```python
from build123d import *

# Parameters (mm, degrees)
SKETCH1_W           = 7.5
SKETCH1_H           = 3.913043478
BOSS_EXTRUDE1_DEPTH = 7.5
SHELL2_T            = -0.75
SKETCH1_4_W         = 7.5
SKETCH1_4_H         = 3.913043478
BOSS_EXTRUDE2_DEPTH = 7.5
HOLE2_D             = 1.6
HOLE2_DEPTH         = 10
HOLE2_CBORE_D       = 3.5
HOLE2_CBORE_DEPTH   = 3
FILLET1_R           = 0.5


with BuildPart() as part:
    # Sketch1 → Boss-Extrude1 (new body)
    with BuildSketch(Plane.XY):
        Polygon((4, 2.086956522), (4, 6), (-4, 6), (-4, 2.086956522), (-11.5, 2.086956522), (-11.5, -2.086956522), (-4, -2.086956522), (-4, -6), (4, -6), (4, -2.086956522), (11.5, -2.086956522), (11.5, 2.086956522), align=None)
        with Locations((-7.75, 4.043478261)):
            Rectangle(SKETCH1_W, SKETCH1_H)
        with Locations((7.75, 4.043478261)):
            Rectangle(SKETCH1_W, SKETCH1_H)
        with Locations((-7.75, -4.043478261)):
            Rectangle(SKETCH1_W, SKETCH1_H)
        with Locations((7.75, -4.043478261)):
            Rectangle(SKETCH1_W, SKETCH1_H)
    extrude(amount=BOSS_EXTRUDE1_DEPTH)

    # Shell2
    shell2_openings = [part.faces().sort_by_distance(p)[0] for p in [
        (0, 0, 7.5),
    ]]
    offset(amount=SHELL2_T, openings=shell2_openings, kind=Kind.INTERSECTION)

    # Sketch1<4> → Boss-Extrude2 (add)
    with BuildSketch(Plane.XY):
        with Locations((7.75, 4.043478261)):
            Rectangle(SKETCH1_4_W, SKETCH1_4_H)
        with Locations((-7.75, 4.043478261)):
            Rectangle(SKETCH1_4_W, SKETCH1_4_H)
        with Locations((-7.75, -4.043478261)):
            Rectangle(SKETCH1_4_W, SKETCH1_4_H)
        with Locations((7.75, -4.043478261)):
            Rectangle(SKETCH1_4_W, SKETCH1_4_H)
    extrude(amount=BOSS_EXTRUDE2_DEPTH)

    # Hole2
    with Locations(Plane(origin=(0, 0, 0), x_dir=(-1, 0, 0), z_dir=(0, 0, -1))):
        with Locations((-9.9, -4), (9.9, 4), (9.9, -4), (-9.9, 4)):
            CounterBoreHole(HOLE2_D / 2, HOLE2_CBORE_D / 2, HOLE2_CBORE_DEPTH, depth=HOLE2_DEPTH)

    # Fillet1
    # the kernel refuses this fillet: 0.5 mm, written as the material it takes off along each edge
    with BuildSketch(Plane(origin=(-11.5, 6, -1.25), x_dir=(1, 0, 0), z_dir=(0, 0, 1)), Plane(origin=(11.5, -6, -1.25), x_dir=(-1, 0, 0), z_dir=(0, 0, 1))) as fillet1_piece_1:
        with BuildLine():
            CenterArc((FILLET1_R, -FILLET1_R), FILLET1_R, 90, 90)
            Line((0, -FILLET1_R), (0, 0))
            Line((0, 0), (FILLET1_R, 0))
        make_face()
    extrude(amount=10, mode=Mode.SUBTRACT)
    with BuildSketch(Plane(origin=(-11.5, 4.541127656, 0), x_dir=(1, 0, 0), z_dir=(0, -1, 0)), Plane(origin=(11.5, 4.541127656, 0), x_dir=(0, 0, 1), z_dir=(0, -1, 0))) as fillet1_piece_2:
        with BuildLine():
            CenterArc((FILLET1_R, FILLET1_R), FILLET1_R, 180, 90)
            Line((0, FILLET1_R), (0, 0))
            Line((0, 0), (FILLET1_R, 0))
        make_face()
    extrude(amount=9.082255312, mode=Mode.SUBTRACT)
    with BuildSketch(Plane(origin=(12.75, 6, 0), x_dir=(0, 0, 1), z_dir=(-1, 0, 0))) as fillet1_piece_3:
        with BuildLine():
            CenterArc((FILLET1_R, -FILLET1_R), FILLET1_R, 90, 90)
            Line((0, -FILLET1_R), (0, 0))
            Line((0, 0), (FILLET1_R, 0))
        make_face()
    extrude(amount=25.5, mode=Mode.SUBTRACT)
    with BuildSketch(Plane(origin=(11.5, 6, -1.25), x_dir=(-1, 0, 0), z_dir=(0, 0, 1)), Plane(origin=(-11.5, -6, -1.25), x_dir=(1, 0, 0), z_dir=(0, 0, 1))) as fillet1_piece_4:
        with BuildLine():
            CenterArc((FILLET1_R, FILLET1_R), FILLET1_R, 180, 90)
            Line((0, FILLET1_R), (0, 0))
            Line((0, 0), (FILLET1_R, 0))
        make_face()
    extrude(amount=10, mode=Mode.SUBTRACT)
    with BuildSketch(Plane(origin=(12.75, -6, 0), x_dir=(0, 0, 1), z_dir=(-1, 0, 0))) as fillet1_piece_5:
        with BuildLine():
            CenterArc((FILLET1_R, FILLET1_R), FILLET1_R, 180, 90)
            Line((0, FILLET1_R), (0, 0))
            Line((0, 0), (FILLET1_R, 0))
        make_face()
    extrude(amount=25.5, mode=Mode.SUBTRACT)


solid = part.part
```
Read the model definition and answer for the solid it produces. Units are mm, in the model's axes. A direction names the side the tool comes from. Give positions to 0.01 mm unless a question says otherwise; leave off trailing zeros. Loops run counter-clockwise (first coordinate to the right, second up) from the corner with the lowest first, then second, coordinate; pieces in that order, holes last.
Item 1: Find the intervals of material crossed by line 1 along Y through (x, z) = (10, 3.75); line 2 along Y through (x, z) = (9.9, 2.05); line 3 along Y through (x, z) = (8.25, 5.25), in increasing order.
Item 2: The mould has two halves that part along X. Classify faces 1 (the flat face through (0, -6, 4)), 2 (the flat face through (11.5, 0, 5)), 3 (the flat face through (0, 5.25, 4)): released by +X, released by -X, zero draft, split by the parting line, or undercut.
Item 3: The part is cut by section A-A (z = 7.25). Write down the section's boundary in (x, y), and give its area (3 significant figures).
Item 4: The part is cut by section C-C (x = 6.25). Write down the section's boundary in (y, z).
Item 5: Each of these flat-tipped pins is pushed along its axis until it touches: pin 1 Ø4 at (x, y) = (-9.9, -4) entering from -Z; pin 2 Ø5 at (x, y) = (-1, -2) entering from +Z. Where does it stop, or does it pass through?
Item 6: The part is cut by section B-B (y = 4). Write down the section's boundary in (x, z).
Item 7: For faces 4 (the cylindrical face through (-9.53, -4.71, 5.28)), 5 (the flat face through (10, 5, 3)), 6 (the flat face through (7, -2.087, 4)), determine the directions among +Z, -Z, +X, -X, +Y, -Y from which every point of the face is accessible in a straight line to the end or side of a thin tool.
Item 8: The part is cut by section D-D (z = 1). Write down the section's boundary in (x, y).
Taken from the geometry:
1. line 1: y = -6 to -4.79, -3.21 to -2.09, 2.09 to 3.21, 4.79 to 6
1. line 2: y = -6 to -5.75, -2.25 to -2.09, 2.09 to 2.25, 5.75 to 6
1. line 3: y = -6 to -2.09, 2.09 to 6
2. face 1: zero draft
2. face 2: released by +X
2. face 3: undercut
3. outline: (-11.5, -5.5) arc R0.5 ccw to (-11, -6) - (11, -6) arc R0.5 ccw to (11.5, -5.5) - (11.5, 5.5) arc R0.5 ccw to (11, 6) - (-11, 6) arc R0.5 ccw to (-11.5, 5.5) - close; hole (-10.75, -2.09) - (-4, -2.09) - (-4, -5.25) - (4, -5.25) - (4, -2.09) - (10.75, -2.09) - (10.75, 2.09) - (4, 2.09) - (4, 5.25) - (-4, 5.25) - (-4, 2.09) - (-10.75, 2.09) - close; hole circle Ø1.6 at (-9.9, -4); hole circle Ø1.6 at (-9.9, 4); hole circle Ø1.6 at (9.9, -4); hole circle Ø1.6 at (9.9, 4)
3. area: 127 mm2
4. outline: (-6, 0.5) arc R0.5 ccw to (-5.5, 0) - (5.5, 0) arc R0.5 ccw to (6, 0.5) - (6, 7.5) - (2.09, 7.5) - (2.09, 0.75) - (-2.09, 0.75) - (-2.09, 7.5) - (-6, 7.5) - close
5. pin 1: stops at z = 0
5. pin 2: stops at z = 0.75
6. outline: (-11.5, 3) - (-10.7, 3) - (-10.7, 7.5) - (-11.5, 7.5) - close; (-9.1, 3) - (-8.15, 3) - (-8.15, 0) - (8.15, 0) - (8.15, 3) - (9.1, 3) - (9.1, 7.5) - (4, 7.5) - (4, 0.75) - (-4, 0.75) - (-4, 7.5) - (-9.1, 7.5) - close; (10.7, 3) - (11.5, 3) - (11.5, 7.5) - (10.7, 7.5) - close
7. face 4: +Z, -Z
7. face 5: -Z
7. face 6: +Z
8. outline: (-11.5, -5.5) arc R0.5 ccw to (-11, -6) - (11, -6) arc R0.5 ccw to (11.5, -5.5) - (11.5, -4.71) arc R1.75 cw (long way) to (11.5, -3.29) - (11.5, 3.29) arc R1.75 cw (long way) to (11.5, 4.71) - (11.5, 5.5) arc R0.5 ccw to (11, 6) - (-11, 6) arc R0.5 ccw to (-11.5, 5.5) - (-11.5, 4.71) arc R1.75 cw (long way) to (-11.5, 3.29) - (-11.5, -3.29) arc R1.75 cw (long way) to (-11.5, -4.71) - close; hole (-10.75, -2.09) - (-4, -2.09) - (-4, -5.25) - (4, -5.25) - (4, -2.09) - (10.75, -2.09) - (10.75, 2.09) - (4, 2.09) - (4, 5.25) - (-4, 5.25) - (-4, 2.09) - (-10.75, 2.09) - close
